Read the model definition and answer for the solid it produces. Units are mm, in the model's axes. Face numbers are marked on the shaded views. A direction names the side the tool comes from. Give positions to 0.01 mm unless a question says otherwise; leave off trailing zeros. Order: outer loops, then holes, each group sorted by start corner. A loop starts at its lowest first (then second) coordinate and runs counter-clockwise, first axis right, second up.
```python
from build123d import *

# Parameters (mm, degrees)
ESQUISSE1_R             = 16
ESQUISSE1_R_2           = 10
BOSS_EXTRU_1_DEPTH      = 7
ESQUISSE2_R             = 14.5
ESQUISSE2_R_2           = 11.5
ENL_V_MAT_EXTRU_1_DEPTH = 0.2
ESQUISSE3_R             = 14.5
ESQUISSE3_R_2           = 11.5
ENL_V_MAT_EXTRU_2_DEPTH = 0.2


with BuildPart() as part:
    # Esquisse1 → Boss.-Extru.1 (new body)
    with BuildSketch(Plane.XY):
        Circle(ESQUISSE1_R)
        Circle(ESQUISSE1_R_2, mode=Mode.SUBTRACT)
    extrude(amount=BOSS_EXTRU_1_DEPTH)

    # Esquisse2 → Enlèv. mat.-Extru.1 (cut)
    with BuildSketch(Plane.XY.offset(7)):
        Circle(ESQUISSE2_R)
        Circle(ESQUISSE2_R_2, mode=Mode.SUBTRACT)
    extrude(amount=-ENL_V_MAT_EXTRU_1_DEPTH, mode=Mode.SUBTRACT)

    # Esquisse3 → Enlèv. mat.-Extru.2 (cut)
    with BuildSketch(Plane(origin=(0, 0, 0), x_dir=(-1, 0, 0), z_dir=(0, 0, -1))):
        Circle(ESQUISSE3_R)
        Circle(ESQUISSE3_R_2, mode=Mode.SUBTRACT)
    extrude(amount=-ENL_V_MAT_EXTRU_2_DEPTH, mode=Mode.SUBTRACT)


solid = part.part
```
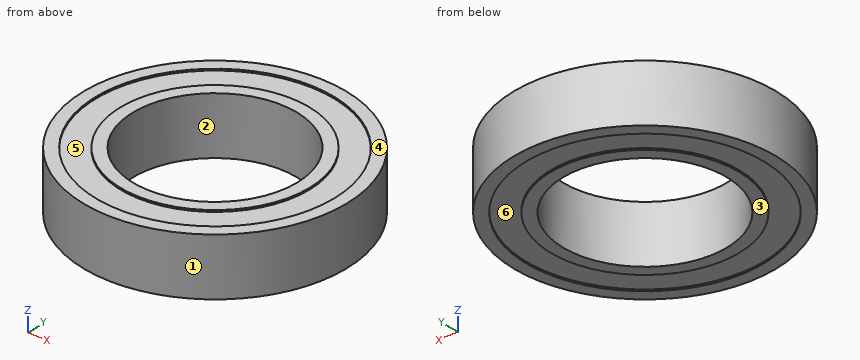
1) Consider L1, parallel to Y at x = 0, z = 0.15; L2, parallel to Z at x = -14, y = -1; L3, parallel to Y at x = -1, z = 6. Determine where each line is inside the solid, lowest interval first.
Final values:
L1: y = -16 to -14.5, -11.5 to -10, 10 to 11.5, 14.5 to 16
L2: z = 0.2 to 6.8
L3: y = -15.97 to -9.95, 9.95 to 15.97
2) Given pin 1 (3 mm diameter, centred on y = -4, z = 1.5, fed in from -X); pin 2 (2 mm diameter, centred on y = 7.5, z = 3, fed in from +X), each flat-ended and moving along its own axis, determine where each tip first touches the part or whether it passes through.
Final values:
pin 1: stops at x = -15.8
pin 2: stops at x = 14.62
3) The part is cut by section A-A on y = 0. Determine the outline of the cut face in (x, z), and give its area (3 significant figures).
Final values:
outline: (-16, 0) - (-14.5, 0) - (-14.5, 0.2) - (-11.5, 0.2) - (-11.5, 0) - (-10, 0) - (-10, 7) - (-11.5, 7) - (-11.5, 6.8) - (-14.5, 6.8) - (-14.5, 7) - (-16, 7) - close; (10, 0) - (11.5, 0) - (11.5, 0.2) - (14.5, 0.2) - (14.5, 0) - (16, 0) - (16, 7) - (14.5, 7) - (14.5, 6.8) - (11.5, 6.8) - (11.5, 7) - (10, 7) - close
area: 81.6 mm2
4) For a pull along Y with two mould halves and no side action, classify the marked faces 1, 2 and 3 as released by +Y, released by -Y, zero draft, split by the parting line, or undercut.
Final values:
face 1: split by the parting line
face 2: undercut
face 3: zero draft
5) The part is cut by section D-D on y = -14. Determine the outline of the cut face in (x, z).
Final values:
outline: (-7.75, 0) - (-3.77, 0) - (-3.77, 0.2) - (3.77, 0.2) - (3.77, 0) - (7.75, 0) - (7.75, 7) - (3.77, 7) - (3.77, 6.8) - (-3.77, 6.8) - (-3.77, 7) - (-7.75, 7) - close
6) A tool of negligible diameter and unlimited length cuts with its end or side. For the marked faces 4, 5 and 6, from which of +Z, -Z, +X, -X, +Y, -Y can it reach the whole face along a straight path? Write none if from no direction.
Final values:
face 4: +Z, +X, -X, +Y, -Y
face 5: +Z
face 6: -Z
7) The part is cut by section C-C on z = 6. Determine the outline of the cut face in (x, y), and give its area (3 significant figures).
Final values:
outline: circle Ø32 at (0, 0); hole circle Ø20 at (0, 0)
area: 490 mm2
